For this review, take the finished solid that the model builds, in its own axes (mm). A direction names the side the tool comes from. Coordinates: 2 decimals unless noted, no trailing zeros. Write each loop counter-clockwise with the first axis right and the second up, starting at its lowest first coordinate (ties: lowest second). Pieces come first, ordered by that corner, then holes. Notation, with made-up numbers: (57, 35.5) - (112, 35.5) arc R24 cw to (112, 72.5) - close; hole circle Ø10 at (-39.75, 47.5). An arc over 180 degrees is marked (long way). Write each question's results on one line, items separated by ' | '.
from build123d import *

# Parameters (mm, degrees)
SKETCH1_W           = 16.600054
SKETCH1_H           = 15
SKETCH1_R           = 1.5
BOSS_EXTRUDE1_DEPTH = 2
BOSS_EXTRUDE2_DEPTH = 1


with BuildPart() as part:
    # Sketch1 → Boss-Extrude1 (new body)
    with BuildSketch(Plane.XY):
        with Locations((12.458065, 13.09497)):
            Rectangle(SKETCH1_W, SKETCH1_H)
        with Locations((6.908038, 13.09497)):
            Circle(SKETCH1_R, mode=Mode.SUBTRACT)
        with BuildLine():
            ThreePointArc((6.908038, 11.09497), (8.908038, 13.09497), (6.908038, 15.09497))
            Line((6.908038, 15.09497), (6.908038, 18.09497))
            Line((6.908038, 18.09497), (18.008092, 18.09497))
            Line((18.008092, 18.09497), (18.008092, 15.09497))
            ThreePointArc((18.008092, 15.09497), (16.008092, 13.09497), (18.008092, 11.09497))
            Line((18.008092, 11.09497), (18.008092, 8.09497))
            Line((18.008092, 8.09497), (6.908038, 8.09497))
            Line((6.908038, 8.09497), (6.908038, 11.09497))
        make_face(mode=Mode.SUBTRACT)
        with Locations((18.008092, 13.09497)):
            Circle(SKETCH1_R, mode=Mode.SUBTRACT)
    extrude(amount=BOSS_EXTRUDE1_DEPTH)

    # Sketch1<25> → Boss-Extrude2 (add)
    with BuildSketch(Plane.XY):
        Polygon((6.908038, 18.09497), (6.908038, 16.59497), (8.866977953, 14.830167817), (10.358845842, 16.48614923), (8.5730461, 18.09497), align=None)
        Polygon((18.008092, 18.09497), (16.3430839, 18.09497), (14.485103938, 16.421122321), (15.943445071, 14.73493677), (18.008092, 16.59497), align=None)
        Polygon((14.485103938, 9.768817679), (16.3430839, 8.09497), (18.008092, 8.09497), (18.008092, 9.59497), (15.943445071, 11.45500323), align=None)
        Polygon((8.866977953, 11.359772183), (6.908038, 9.59497), (6.908038, 8.09497), (8.5730461, 8.09497), (10.358845842, 9.70379077), align=None)
    extrude(amount=BOSS_EXTRUDE2_DEPTH)


solid = part.part
Q1. Take a section at D-D on z = 1.55. State the section outline as (x, y) points, plus the area to 3 significant figures.
Results found:
outline: (4.16, 5.59) - (20.76, 5.59) - (20.76, 20.59) - (4.16, 20.59) - close; hole circle Ø3 at (6.91, 13.09); hole (6.91, 8.09) - (18.01, 8.09) - (18.01, 11.09) arc R2 cw to (18.01, 15.09) - (18.01, 18.09) - (6.91, 18.09) - (6.91, 15.09) arc R2 cw to (6.91, 11.09) - close; hole circle Ø3 at (18.01, 13.09) | area: 136 mm2
Q2. Take a section at B-B on y = 13.5. State the section outline as (x, z) points.
Results found:
outline: (4.16, 0) - (5.46, 0) - (5.46, 2) - (4.16, 2) - close; (8.35, 0) - (8.87, 0) - (8.87, 2) - (8.35, 2) - close; (16.05, 0) - (16.56, 0) - (16.56, 2) - (16.05, 2) - close; (19.45, 0) - (20.76, 0) - (20.76, 2) - (19.45, 2) - close
Q3. Take a section at A-A on x = 11.75. State the section outline as (y, z) points.
Results found:
outline: (5.59, 0) - (8.09, 0) - (8.09, 2) - (5.59, 2) - close; (18.09, 0) - (20.59, 0) - (20.59, 2) - (18.09, 2) - close
Q4. Wall thickness on line 1 along Y through (x, z) = (10.5, 1.7); line 2 along Y through (x, z) = (8.25, 0.15); line 3 along Y through (x, z) = (8, 1.65): over which ranges is each line inside the solid? List them lowest first. Write a range as from..to.
Results found:
line 1: 5.59..8.09, 18.09..20.59 | line 2: 5.59..10.8, 11.61..12.42, 13.77..14.58, 15.39..20.59 | line 3: 5.59..8.09, 11.42..12.07, 14.12..14.77, 18.09..20.59
Q5. Take a section at C-C on x = 8. State the section outline as (y, z) points, plus the area to 3 significant figures.
Results found:
outline: (5.59, 0) - (10.58, 0) - (10.58, 1) - (8.09, 1) - (8.09, 2) - (5.59, 2) - close; (11.42, 0) - (12.07, 0) - (12.07, 2) - (11.42, 2) - close; (14.12, 0) - (14.77, 0) - (14.77, 2) - (14.12, 2) - close; (15.61, 0) - (20.59, 0) - (20.59, 2) - (18.09, 2) - (18.09, 1) - (15.61, 1) - close | area: 17.6 mm2
Q6. For faces 3 (the face through (18.008, 10, 1)), 4 (the face through (9.602, 15.647, 0.493)), list the 3-axis set-ups (+Z, -Z, +X, -X, +Y, -Y) from which the entire face can be reached by the end or side of a thin tool; tool diameter is ignored.
Results found:
face 3: +Z | face 4: +Z, -Z
Q7. Mouldability with a two-part tool opening along Y and no side actions: class faces 1 (the face through (12, 5.595, 1)), 2 (the face through (15.43, 17.27, 0.49)) as pulls with the +Y half, pulls with the -Y half, needs draft (parallel to the pull), parting line crosses it, or undercut.
Results found:
face 1: pulls with the -Y half | face 2: undercut
Q8. For pin 1 (2.5 mm diameter, centred on x = 6.91, y = 13.09, fed in from +Z); pin 2 (1 mm diameter, centred on x = 16, y = 10, fed in from +Z), all flat-tipped, find the tip position at first contact; note any pin that passes through.
Results found:
pin 1: through | pin 2: z = 1
